Geometry: final body of the model. Coordinates: model frame, mm. Face numbers are marked on the shaded views. A direction names the side the tool comes from. Coordinates: 2 decimals unless noted, no trailing zeros. Order: outer loops, then holes, each group sorted by start corner. A loop starts at its lowest first (then second) coordinate and runs counter-clockwise, first axis right, second up. Notation, with made-up numbers: M 69,63 L 126,63 A28 cw 126,82 Z; hole C -33.5,-9.75 d5. An arc over 180 degrees is marked long. Write item = value, one per line.
from build123d import *

# Parameters (mm, degrees)
F1_DEPTH = 63.5
F3_DEPTH = 6.35


with BuildPart() as f1:
    # F0 (on Top) → F1 (new body)
    with BuildSketch(Plane.XY):
        with BuildLine():
            Line((139.7, 114.3), (-139.7, 114.3))
            ThreePointArc((-139.7, 114.3), (-148.680256, 110.580256), (-152.4, 101.6))
            Line((-152.4, 101.6), (-152.4, -101.6))
            ThreePointArc((-152.4, -101.6), (-148.680256, -110.580256), (-139.7, -114.3))
            Line((-139.7, -114.3), (139.7, -114.3))
            ThreePointArc((139.7, -114.3), (148.680256, -110.580256), (152.4, -101.6))
            Line((152.4, -101.6), (152.4, 101.6))
            ThreePointArc((152.4, 101.6), (148.680256, 110.580256), (139.7, 114.3))
        make_face()
        with BuildLine():
            ThreePointArc((-146.05, 101.6), (-144.190128, 106.090128), (-139.7, 107.95))
            Line((-139.7, 107.95), (139.7, 107.95))
            ThreePointArc((139.7, 107.95), (144.190128, 106.090128), (146.05, 101.6))
            Line((146.05, 101.6), (146.05, -101.6))
            ThreePointArc((146.05, -101.6), (144.190128, -106.090128), (139.7, -107.95))
            Line((139.7, -107.95), (-139.7, -107.95))
            ThreePointArc((-139.7, -107.95), (-144.190128, -106.090128), (-146.05, -101.6))
            Line((-146.05, -101.6), (-146.05, 101.6))
        make_face(mode=Mode.SUBTRACT)
    extrude(amount=F1_DEPTH)

    # F2 (on Top) → F3 (join)
    with BuildSketch(Plane.XY):
        with BuildLine():
            ThreePointArc((-152.4, -101.6), (-148.680256, -110.580256), (-139.7, -114.3))
            Line((-139.7, -114.3), (139.7, -114.3))
            ThreePointArc((139.7, -114.3), (148.680256, -110.580256), (152.4, -101.6))
            Line((152.4, -101.6), (152.4, 101.6))
            ThreePointArc((152.4, 101.6), (148.680256, 110.580256), (139.7, 114.3))
            Line((139.7, 114.3), (-139.7, 114.3))
            ThreePointArc((-139.7, 114.3), (-148.680256, 110.580256), (-152.4, 101.6))
            Line((-152.4, 101.6), (-152.4, -101.6))
        make_face()
    extrude(amount=-F3_DEPTH)


solid = f1.part
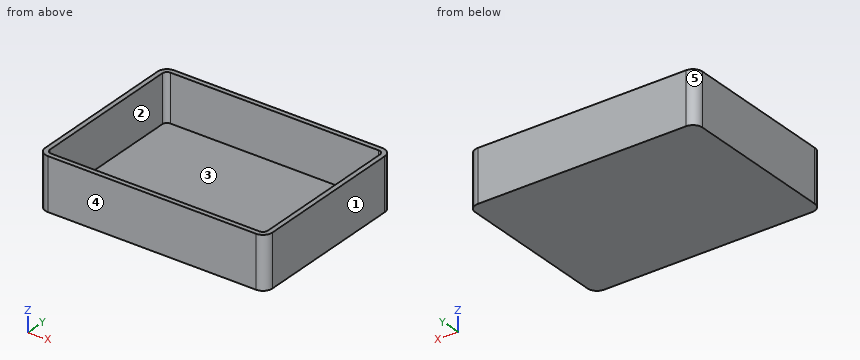
1) Section B-B, the plane y = -66. Return loops of the section in (x, z).
Numbers:
outline = M -152.4,-6.35 L 152.4,-6.35 L 152.4,63.5 L 146.05,63.5 L 146.05,0 L -146.05,0 L -146.05,63.5 L -152.4,63.5 Z
2) Section A-A, the plane x = -25.5. Return loops of the section in (y, z).
Numbers:
outline = M -114.3,-6.35 L 114.3,-6.35 L 114.3,63.5 L 107.95,63.5 L 107.95,0 L -107.95,0 L -107.95,63.5 L -114.3,63.5 Z
3) Line query: L1, parallel to Y at x = 14, z = 30.5; L2, parallel to X at y = 67, z = 26; L3, parallel to Z at x = -70.5, y = -80.5. Output: solid intervals per line, ascending.
Numbers:
L1 = -114.3 to -107.95, 107.95 to 114.3
L2 = -152.4 to -146.05, 146.05 to 152.4
L3 = -6.35 to 0
4) Mould query, pull axis Y, two halves, no side actions, for the marked faces 3, 4 and 5. Classes: pulls with the +Y half, pulls with the -Y half, needs draft (parallel to the pull), parting line crosses it, or undercut.
Numbers:
face_3 = undercut
face_4 = pulls with the -Y half
face_5 = pulls with the +Y half
5) Section C-C, the plane z = 40. Return loops of the section in (x, y), and give its area (3 significant figures).
Numbers:
outline = M -152.4,-101.6 A12.7 ccw -139.7,-114.3 L 139.7,-114.3 A12.7 ccw 152.4,-101.6 L 152.4,101.6 A12.7 ccw 139.7,114.3 L -139.7,114.3 A12.7 ccw -152.4,101.6 Z; hole M -146.05,-101.6 A6.35 ccw -139.7,-107.95 L 139.7,-107.95 A6.35 ccw 146.05,-101.6 L 146.05,101.6 A6.35 ccw 139.7,107.95 L -139.7,107.95 A6.35 ccw -146.05,101.6 Z
area = 6,510 mm²
6) Set-up query: the marked faces 1 and 2. Return all of +Z, -Z, +X, -X, +Y, -Y with unobstructed straight access to the full face (end or side cutting, diameter ignored); none if empty.
Numbers:
face_1 = +Z, -Z, +X, +Y, -Y
face_2 = +Z
